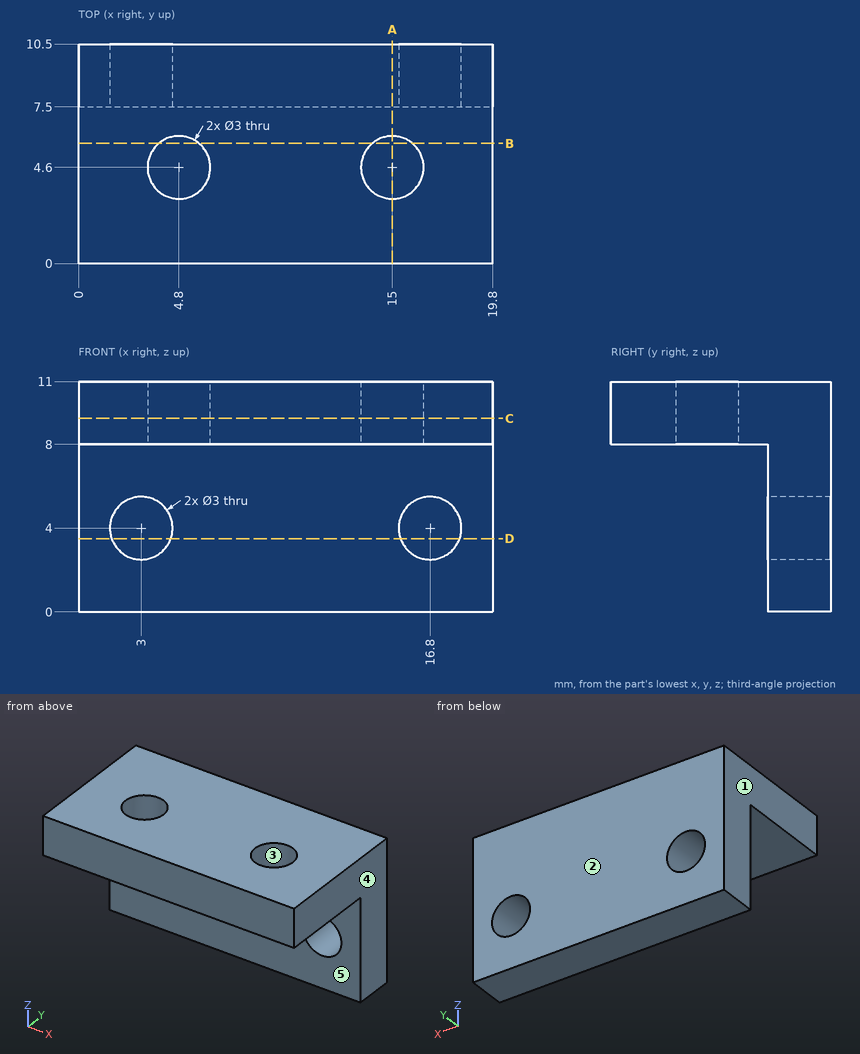
Verification items for this drawing (mm, ordinates from the low corner). A direction names the side the tool comes from. Give positions to 0.01 mm unless a question says otherwise; leave off trailing zeros. Loops run counter-clockwise (first coordinate to the right, second up) from the corner with the lowest first, then second, coordinate; pieces in that order, holes last. Notation, with made-up numbers: M 69.5,59 L 76.5,59 A24 ccw 76.5,95 Z; hole C 32,14 d3. An arc over 180 degrees is marked long. Write item = value, one per line. Start each with the question number.
1. Thickness scan on probe 1 along Y at (x, z) = (4.8, 10.4); probe 2 along X at (y, z) = (8, 2.75); probe 3 along Z at (x, y) = (16.8, 8.8). Record the ranges inside material, lowest first.
2. Tool access check on the marked faces 4 and 5. Record the directions out of +Z, -Z, +X, -X, +Y, -Y that give a thin tool (end or side, any length) a straight path to the whole face; none if there is none.
3. Section check A-A, the plane x = 15. Enter the section's corners in (y, z).
4. Section check B-B, the plane y = 5.75. Enter the section's corners in (x, z), plus the area to 3 significant figures.
5. Draft check along X on the marked faces 1, 2 and 3. Enter one of: +X half, -X half, draft (parallel to the pull), parting line (faces both ways), or undercut.
6. Go/stop test with flat-tipped pins: P1, Ø4, axis at x = 4, z = 5, coming from the -Y side; P2, Ø2, axis at x = 10.5, y = 2, coming from the -Z side. Record where each tip stops, or that it passes through.
7. Section check C-C, the plane z = 9.25. Enter the section's corners in (x, y).
8. Section check D-D, the plane z = 3.5. Enter the section's corners in (x, y).
Values follow:
q1.probe_1 = 0 to 3.1, 6.1 to 10.5
q1.probe_2 = 0 to 2.17, 3.83 to 15.97, 17.63 to 19.8
q1.probe_3 = 0 to 2.5, 5.5 to 11
q2.face_4 = +Z, -Z, +X, +Y, -Y
q2.face_5 = -Z, +X, -X, -Y
q3.outline = M 0,8 L 3.1,8 L 3.1,11 L 0,11 Z; M 6.1,8 L 7.5,8 L 7.5,0 L 10.5,0 L 10.5,11 L 6.1,11 Z
q4.outline = M 0,8 L 3.84,8 L 3.84,11 L 0,11 Z; M 5.76,8 L 14.04,8 L 14.04,11 L 5.76,11 Z; M 15.96,8 L 19.8,8 L 19.8,11 L 15.96,11 Z
q4.area = 47.8 mm^2
q5.face_1 = -X half
q5.face_2 = draft
q5.face_3 = undercut
q6.P1 = 7.5
q6.P2 = 8
q7.outline = M 0,0 L 19.8,0 L 19.8,10.5 L 0,10.5 Z; hole C 4.8,4.6 d3; hole C 15,4.6 d3
q8.outline = M 0,7.5 L 1.59,7.5 L 1.59,10.5 L 0,10.5 Z; M 4.41,7.5 L 15.39,7.5 L 15.39,10.5 L 4.41,10.5 Z; M 18.21,7.5 L 19.8,7.5 L 19.8,10.5 L 18.21,10.5 Z
